```python
from build123d import *

# Parameters (mm, degrees)
SKETCH1_W           = 40.6
SKETCH1_H           = 39.25
BOSS_EXTRUDE1_DEPTH = 10.08
BOSS_EXTRUDE2_DEPTH = 2.4
SKETCH3_W           = 6.4
SKETCH3_H           = 4.1
BOSS_EXTRUDE3_DEPTH = 6
SKETCH4_R           = 2.87
BOSS_EXTRUDE4_DEPTH = 3.9


with BuildPart() as part:
    # Sketch1 → Boss-Extrude1 (new, symmetric)
    with BuildSketch(Plane(origin=(0, 0, 0), x_dir=(0, 0, -1), z_dir=(1, 0, 0))):
        with Locations((0, 19.625)):
            Rectangle(SKETCH1_W, SKETCH1_H)
    extrude(amount=BOSS_EXTRUDE1_DEPTH, both=True)

    # Sketch2 → Boss-Extrude2 (add)
    with BuildSketch(Plane(origin=(0, 29.14, 0), x_dir=(1, 0, 0), z_dir=(0, 1, 0))):
        with BuildLine():
            Line((-10.08, -20.3), (10.08, -20.3))
            Line((10.08, -20.3), (10.08, -27.13))
            Line((10.08, -27.13), (6.124613606, -27.13))
            Line((6.124613606, -27.13), (6.124613606, -26.094160296))
            ThreePointArc((6.124613606, -26.094160296), (4.925, -22.05), (3.725386394, -26.094160296))
            Line((3.725386394, -26.094160296), (3.725386394, -27.13))
            Line((3.725386394, -27.13), (-3.725386394, -27.13))
            Line((-3.725386394, -27.13), (-3.725386394, -26.094160296))
            ThreePointArc((-3.725386394, -26.094160296), (-4.925, -22.05), (-6.124613606, -26.094160296))
            Line((-6.124613606, -26.094160296), (-6.124613606, -27.13))
            Line((-6.124613606, -27.13), (-10.08, -27.13))
            Line((-10.08, -27.13), (-10.08, -20.3))
        make_face()
    boss_extrude2 = extrude(amount=-BOSS_EXTRUDE2_DEPTH)

    # Mirror1: Boss-Extrude2 across plane
    add(boss_extrude2.mirror(Plane.XY))

    # Sketch3 → Boss-Extrude3 (add)
    with BuildSketch(Plane(origin=(0, 0, -20.3), x_dir=(-1, 0, 0), z_dir=(0, 0, -1))):
        with Locations((0, 5.524349408)):
            Rectangle(SKETCH3_W, SKETCH3_H)
    extrude(amount=BOSS_EXTRUDE3_DEPTH)

    # Sketch4 → Boss-Extrude4 (add)
    with BuildSketch(Plane(origin=(0, 39.25, 0), x_dir=(1, 0, 0), z_dir=(0, 1, 0))):
        with Locations(Location((0, 12, 0), (0, 0, 90))):
            Circle(SKETCH4_R)
    extrude(amount=BOSS_EXTRUDE4_DEPTH)


solid = part.part
```
Model file for the job. Use its own axes, mm. A direction names the side the tool comes from. Coordinates: 2 decimals unless noted, no trailing zeros. Loops run counter-clockwise (first coordinate to the right, second up) from the corner with the lowest first, then second, coordinate; pieces in that order, holes last. Notation, with made-up numbers: (1, -27.5) - (27, -27.5) arc R7 ccw to (27, -17.5) - close; hole circle Ø4 at (-33, -19.5). An arc over 180 degrees is marked (long way). Answer as a JSON object with one key per item and string values. Group by question number.
(1) Cut at C-C (x = 0). Give the cut face in (y, z).
(2) Tool access for faces 1 (the face through (0, 6, -26.3)), 2 (the face through (5, 27.96, -22.05)), 3 (the face through (0, 29.14, 24)), 4 (the face through (3.2, 5, -23)), 5 (the face through (-3.2, 5, -23)): list every direction of +Z, -Z, +X, -X, +Y, -Y with a clear straight run to the whole face (end or side of a thin tool).
(3) Probe line 1 along X through (y, z) = (27.7, -24.25) (3 decimals); line 2 along Z through (x, y) = (6.25, 28); line 3 along Z through (x, y) = (1, 25). List the from-to ranges inside material, lowest first.
(4) Flat gauge pins, fed straight in: pin 1 (2 mm diameter, centred on x = -7, y = 32.5, fed in from -Z); pin 2 (10 mm diameter, centred on x = -3, y = 6.5, fed in from -Z); pin 3 (8 mm diameter, centred on x = -5, y = 33.5, fed in from +Z). Where does each tip first touch, or does it go through?
(5) Cut at B-B (z = 24.25). Give the cut face in (x, y) (3 decimals), then the cut area to 3 significant figures.
(6) Two-plate mould, pull along Y, no slides. Class faces 6 (the face through (0, 26.74, -24)), 7 (the face through (-4.85, 27.96, -22.05)), 8 (the face through (0, 29.14, -24)): released by +Y, released by -Y, zero draft, split by the parting line, or undercut.
(7) Cut at D-D (z = -12). Give the cut face in (x, y).
(8) Cut at A-A (z = -24.25). Give the cut face in (x, y) (3 decimals), then the cut area to 3 significant figures.
Geometry says:
{
 "1": {"outline": "(0, -20.3) - (3.47, -20.3) - (3.47, -26.3) - (7.57, -26.3) - (7.57, -20.3) - (26.74, -20.3) - (26.74, -27.13) - (29.14, -27.13) - (29.14, -20.3) - (39.25, -20.3) - (39.25, -14.87) - (43.15, -14.87) - (43.15, -9.13) - (39.25, -9.13) - (39.25, 20.3) - (29.14, 20.3) - (29.14, 27.13) - (26.74, 27.13) - (26.74, 20.3) - (0, 20.3) - close"},
 "2": {"face 1": "-Z, +X, -X, -Y", "face 2": "+Y", "face 3": "+Z, +X, -X, +Y", "face 4": "-Z, +X, -Y", "face 5": "-Z, -X, -Y"},
 "3": {"line 1": "x = -10.08 to -7.125, -2.725 to 2.725, 7.125 to 10.08", "line 2": "z = -27.13 to -26.01, -22.49 to 22.49, 26.01 to 27.13", "line 3": "z = -20.3 to 20.3"},
 "4": {"pin 1": "stops at z = -20.3", "pin 2": "stops at z = -26.3", "pin 3": "stops at z = 20.3"},
 "5": {"outline": "(-10.08, 26.74) - (-7.125, 26.74) - (-7.125, 29.14) - (-10.08, 29.14) - close; (-2.725, 26.74) - (2.725, 26.74) - (2.725, 29.14) - (-2.725, 29.14) - close; (7.125, 26.74) - (10.08, 26.74) - (10.08, 29.14) - (7.125, 29.14) - close", "area": "27.3 mm^2"},
 "6": {"face 6": "undercut", "face 7": "zero draft", "face 8": "released by +Y"},
 "7": {"outline": "(-10.08, 0) - (10.08, 0) - (10.08, 39.25) - (2.87, 39.25) - (2.87, 43.15) - (-2.87, 43.15) - (-2.87, 39.25) - (-10.08, 39.25) - close"},
 "8": {"outline": "(-10.08, 26.74) - (-7.125, 26.74) - (-7.125, 29.14) - (-10.08, 29.14) - close; (-3.2, 3.474) - (3.2, 3.474) - (3.2, 7.574) - (-3.2, 7.574) - close; (-2.725, 26.74) - (2.725, 26.74) - (2.725, 29.14) - (-2.725, 29.14) - close; (7.125, 26.74) - (10.08, 26.74) - (10.08, 29.14) - (7.125, 29.14) - close", "area": "53.5 mm^2"}
}
